Verification items for this drawing (mm, ordinates from the low corner). A direction names the side the tool comes from. Give positions to 0.01 mm unless a question says otherwise; leave off trailing zeros. Loops run counter-clockwise (first coordinate to the right, second up) from the corner with the lowest first, then second, coordinate; pieces in that order, holes last. Notation, with made-up numbers: (44, 62) -> (50, 62) arc R25 cw to (50, 84) -> close; hole circle Ø9 at (89.25, 31). An arc over 180 degrees is marked (long way). Write each question's results on one line, items separated by ' | '. Start each with the question number.
1) Sectioned sample at C-C on x = 51. Record the cut outline in (y, z), then the cut area to 3 significant figures.
2) Set-up check for the marked faces 4 and 5: record each of +Z, -Z, +X, -X, +Y, -Y from which the full face is reachable in a straight line by a thin tool's end or side.
3) Draft check along X on the marked faces 1, 2 and 3. Enter one of: pulls with the +X half, pulls with the -X half, needs draft (parallel to the pull), parting line crosses it, or undercut.
4) Scan lines: line 1 (X direction, y = 7.75, z = 39.5); line 2 (Z direction, x = 60.5, y = 8.75). Record each from-to range of solid material in increasing order. Write a range as from..to.
5) Sectioned sample at B-B on y = 2.5. Record the cut outline in (x, z).
6) Sectioned sample at A-A on z = 32. Record the cut outline in (x, y), then the cut area to 3 significant figures.
7) Depth check by flat-ended pin: pin 1 (9 mm diameter, centred on y = 6.5, z = 22, fed in from -X). Enter the tip coordinate at first touch or a pass-through.
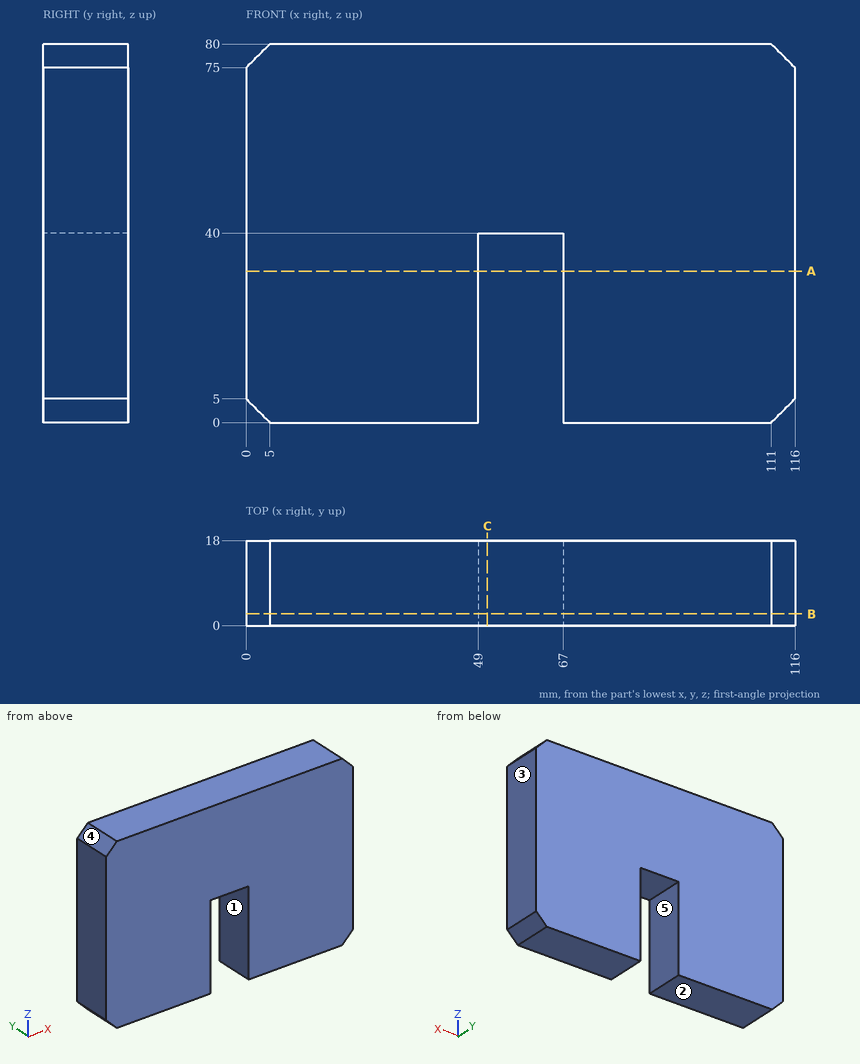
Result:
1) outline: (0, 40) -> (18, 40) -> (18, 80) -> (0, 80) -> close | area: 720 mm^2
2) face 4: +Z, -X, +Y, -Y | face 5: -Z, +Y, -Y
3) face 1: undercut | face 2: needs draft | face 3: pulls with the +X half
4) line 1: 0..49, 67..116 | line 2: 40..80
5) outline: (0, 5) -> (5, 0) -> (49, 0) -> (49, 40) -> (67, 40) -> (67, 0) -> (111, 0) -> (116, 5) -> (116, 75) -> (111, 80) -> (5, 80) -> (0, 75) -> close
6) outline: (0, 0) -> (49, 0) -> (49, 18) -> (0, 18) -> close; (67, 0) -> (116, 0) -> (116, 18) -> (67, 18) -> close | area: 1,760 mm^2
7) pin 1: x = 0
